from build123d import *

# Parameters (mm, degrees)
SALIENTE_EXTRUIR1_DEPTH      = 7
CROQUIS5_R                   = 1.6
CORTAR_EXTRUIR2_DEPTH        = 13.9
CROQUIS6_R                   = 2.75
CORTAR_EXTRUIR3_DEPTH        = 3
SALIENTE_EXTRUIR2_DEPTH      = 5
SALIENTE_EXTRUIR2_DEPTH_BACK = 12
CROQUIS8_R                   = 1.45
CORTAR_EXTRUIR4_DEPTH        = 10
CROQUIS9_W                   = 2
CROQUIS9_H                   = 0.75
CORTAR_EXTRUIR5_DEPTH        = 10


with BuildPart() as part:
    # Croquis1 → Saliente-Extruir1 (new body)
    with BuildSketch(Plane.XY):
        Polygon((0, 0), (4, 0), (4, -4), (7, -4), (7, 0), (7, 13.75), (10.5, 13.75), (10.5, 15.75), (9.5, 15.75), (9.5, 16.5), (7, 16.5), (0, 16.5), (0, 9.5), (-7, 9.5), (-7, 0), align=None)
    extrude(amount=SALIENTE_EXTRUIR1_DEPTH)

    # Croquis5 → Cortar-Extruir2 (cut)
    with BuildSketch(Plane(origin=(0, 9.5, 0), x_dir=(1, 0, 0), z_dir=(0, 1, 0))):
        with Locations(Location((-3.5, -3.5, 0), (0, 0, 180))):
            Circle(CROQUIS5_R)
    extrude(amount=-CORTAR_EXTRUIR2_DEPTH, mode=Mode.SUBTRACT)

    # Croquis6 → Cortar-Extruir3 (cut)
    with BuildSketch(Plane(origin=(0, 9.5, 0), x_dir=(1, 0, 0), z_dir=(0, 1, 0))):
        with Locations(Location((-3.5, -3.5, 0), (0, 0, 180))):
            Circle(CROQUIS6_R)
    extrude(amount=-CORTAR_EXTRUIR3_DEPTH, mode=Mode.SUBTRACT)

    # Croquis7 → Saliente-Extruir2 (add, two sides: drawn at the far end of the back side and taken through both)
    with BuildSketch(Plane.XY.offset(7).offset(-SALIENTE_EXTRUIR2_DEPTH_BACK)):
        Polygon((0, 16.5), (0, 0), (7, 0), (7, 13.75), (10.5, 13.75), (10.5, 15.75), (9.5, 15.75), (9.5, 16.5), align=None)
    extrude(amount=SALIENTE_EXTRUIR2_DEPTH + SALIENTE_EXTRUIR2_DEPTH_BACK)

    # Croquis8 → Cortar-Extruir4 (cut)
    with BuildSketch(Plane(origin=(0, 16.5, 0), x_dir=(1, 0, 0), z_dir=(0, 1, 0))):
        with Locations(Location((3.5, 1.8, 0), (0, 0, 270))):
            Circle(CROQUIS8_R)
        with Locations(Location((3.5, -8.8, 0), (0, 0, 90))):
            Circle(CROQUIS8_R)
    extrude(amount=-CORTAR_EXTRUIR4_DEPTH, mode=Mode.SUBTRACT)

    # Croquis9 → Cortar-Extruir5 (cut)
    with BuildSketch(Plane(origin=(9.5, 0, 0), x_dir=(0, 0, -1), z_dir=(1, 0, 0))):
        with Locations((-3.5, 16.125)):
            Rectangle(CROQUIS9_W, CROQUIS9_H)
    extrude(amount=-CORTAR_EXTRUIR5_DEPTH, mode=Mode.SUBTRACT)


solid = part.part
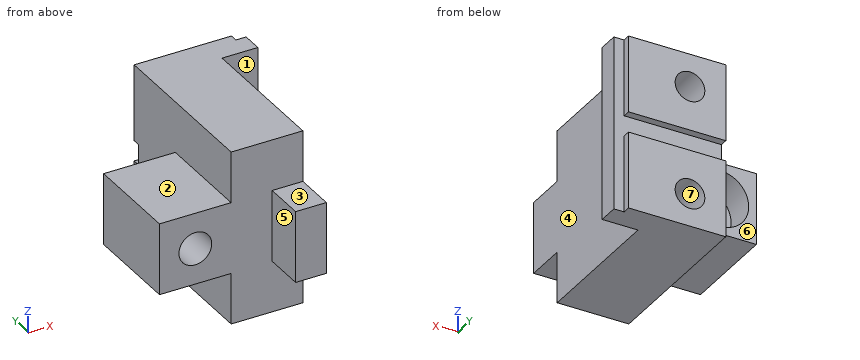
For this review, take the finished solid that the model builds, in its own axes (mm). Face numbers are marked on the shaded views. A direction names the side the tool comes from. Give positions to 0.01 mm unless a question says otherwise; leave off trailing zeros. Order: outer loops, then holes, each group sorted by start corner. A loop starts at its lowest first (then second) coordinate and runs counter-clockwise, first axis right, second up. Notation, with made-up numbers: (47, 65.5) - (80, 65.5) arc R5 ccw to (80, 71.5) - close; hole circle Ø9 at (22, 27.5). An arc over 180 degrees is marked (long way). Answer as a JSON object with one key per item and string values. Group by question number.
Item 1: Take a section at C-C on y = 9. Give the boundary of the cut face in (x, z).
Item 2: Take a section at D-D on y = 1. Give the boundary of the cut face in (x, z), and give its area (3 significant figures).
Item 3: Wall thickness on line 1 along X through (y, z) = (9.75, -1.8); line 2 along Z through (x, y) = (-3.5, 7.7); line 3 along X through (y, z) = (-2, 3.5): over which ranges is each line inside the solid? List them lowest first.
Item 4: Clearance check with flat-ended pins moving along their axes: pin 1 Ø1.8 at (x, z) = (9.5, 6) entering from -Y; pin 2 Ø3.5 at (x, y) = (5, -2) entering from -Z; pin 3 Ø1.5 at (y, z) = (7, 5.5) entering from +X. State where each tip first meets the part, or that it passes through.
Item 5: Take a section at B-B on x = -3.5. Give the boundary of the cut face in (y, z), and give its area (3 significant figures).
Item 6: Machinability: for the marked faces 1, 2 and 3, which of the approach directions +Z, -Z, +X, -X, +Y, -Y give a long, thin tool a straight path to every point of the face, cutting with its end or side? Answer none if there is none.
Item 7: Take a section at A-A on z = 3.5. Give the boundary of the cut face in (x, y).
Item 8: Draft analysis for pull direction X (two halves, no side actions). For the marked faces 4, 5, 6 and 7, state which applies: pulls with the +X half, pulls with the -X half, needs draft (parallel to the pull), parting line crosses it, or undercut.
Reported:
{
 "1": {"outline": "(-7, 0) - (0, 0) - (0, -5) - (7, -5) - (7, 12) - (0, 12) - (0, 7) - (-7, 7) - close; hole circle Ø5.5 at (-3.5, 3.5); hole circle Ø2.9 at (3.5, -1.8); hole circle Ø2.9 at (3.5, 8.8)"},
 "2": {"outline": "(-7, 0) - (0, 0) - (0, -5) - (7, -5) - (7, 12) - (0, 12) - (0, 7) - (-7, 7) - close; hole circle Ø3.2 at (-3.5, 3.5)", "area": "160 mm^2"},
 "3": {"line 1": "0 to 2.05, 4.95 to 7", "line 2": "0 to 0.75, 6.25 to 7", "line 3": "4 to 7"},
 "4": {"pin 1": "y = 13.75", "pin 2": "z = 0", "pin 3": "x = 7"},
 "5": {"outline": "(0, 0) - (9.5, 0) - (9.5, 0.75) - (6.5, 0.75) - (6.5, 1.9) - (0, 1.9) - close; (0, 5.1) - (6.5, 5.1) - (6.5, 6.25) - (9.5, 6.25) - (9.5, 7) - (0, 7) - close", "area": "29.2 mm^2"},
 "6": {"face 1": "+Z, -Z, +X, -Y", "face 2": "+Z, -X, +Y, -Y", "face 3": "+Z, +X, -X, -Y"},
 "7": {"outline": "(-7, 0) - (-5.1, 0) - (-5.1, 6.5) - (-6.25, 6.5) - (-6.25, 9.5) - (-7, 9.5) - close; (-1.9, 0) - (4, 0) - (4, -4) - (7, -4) - (7, 13.75) - (10.5, 13.75) - (10.5, 15.75) - (0, 15.75) - (0, 9.5) - (-0.75, 9.5) - (-0.75, 6.5) - (-1.9, 6.5) - close"},
 "8": {"face 4": "pulls with the +X half", "face 5": "pulls with the -X half", "face 6": "needs draft", "face 7": "undercut"}
}
